For this review, take the finished solid that the model builds, in its own axes (mm). A direction names the side the tool comes from. Coordinates: 2 decimals unless noted, no trailing zeros. Write each loop counter-clockwise with the first axis right and the second up, starting at its lowest first coordinate (ties: lowest second). Pieces come first, ordered by that corner, then holes.
Autodesk Inventor part; units mm, degrees
ref_plane "YZ Plane" through (0, 0, 0) normal (1, 0, 0) x (0, 1, 0)
ref_plane "XZ Plane" through (0, 0, 0) normal (0, 1, 0) x (-1, 0, 0)
ref_plane "XY Plane" through (0, 0, 0) normal (0, 0, 1) x (1, 0, 0)
sketch "Szkic1" plane through (0, 0, 0) normal (0, 1, 0) x (-1, 0, 0)
  circle A0 centre (0, 0) radius 19.62 construction
  line L0 (0, 0) -> (-19.62, 0) construction
  circle A1 centre (0, 0) radius 22.5 construction
  circle A2 centre (-19.3219, 3.407) radius 1.75
  circle A3 centre (-19.3219, -3.407) radius 1.75
  circle A4 centre (6.7104, 18.4368) radius 1.75
  circle A5 centre (12.6115, 15.0298) radius 1.75
  circle A6 centre (12.6115, -15.0298) radius 1.75
  circle A7 centre (6.7104, -18.4368) radius 1.75
  circle A8 centre (0, 0) radius 35
  circle A9 centre (-19.3219, 3.407) radius 3.25
  circle A10 centre (-19.3219, -3.407) radius 3.25
  circle A11 centre (6.7104, -18.4368) radius 3.25
  circle A12 centre (12.6115, -15.0298) radius 3.25
  circle A13 centre (12.6115, 15.0298) radius 3.25
  circle A14 centre (6.7104, 18.4368) radius 3.25
  line L1 (14.2365, 17.8444) -> (8.3354, 21.2514)
  line L2 (10.9865, 12.2152) -> (5.0854, 15.6222)
  line L3 (-16.0719, 3.407) -> (-16.0719, -3.407)
  line L4 (14.2365, -17.8444) -> (8.3354, -21.2514)
  line L5 (10.9865, -12.2152) -> (5.0854, -15.6222)
  line L6 (-22.5719, -3.407) -> (-22.5719, 3.407)
  line L7 (-40, 35) -> (40, 35)
  line L8 (40, 35) -> (40, -35)
  line L9 (40, -35) -> (-40, -35)
  line L10 (-40, -35) -> (-40, 35)
  line L11 (-40, 35) -> (40, -35) construction
  line L12 (40, 35) -> (-40, -35) construction
  line L13 (0, -35) -> (0, 35)
  line L14 (40, 0) -> (-40, 0)
  line L15 (56, 0) -> (-56, 0)
  point P0 (0, -35)
  point P1 (0, 35)
  point P2 (35, 0)
  point P3 (-35, 0)
  dimension "d0" = 39.24
  dimension "d1" = 3.5
  dimension "d2" = 20
  dimension "d5" = 360
  dimension "d7" = 45
  dimension "d8" = 70
  dimension "d12" = 6.5
  dimension "d15" = 360
  dimension "d27" = 80
  dimension "d28" = 70
revolve "Obrót2" add sketch "Szkic1" angle 180 about axis through (-10, 0, 0) along (-1, 0, 0) picked at (16.0586, 3.9431) contours A2 | A4 | A5 | L14 L13 A8 | A8 L7 L8 L14 | L13 L14 L3 A9 L6 A8 | A8 L14 L10 L7 | L14 L6 A9 L3 | A9 | A13 | A13 L2 A14 L1 | A14
extrude "Wyciągnięcie proste1" cut sketch "Szkic1" along normal through all contours A2 | A3 | A4 | A5 | A6 | A7 | L14 L6 A9 L3 | L3 A10 L6 L14 | A9 | A10 | A11 | A11 L5 A12 L4 | A12 | A13 | A13 L2 A14 L1 | A14
extrude "Wyciągnięcie proste2" add sketch "Szkic1" along normal blind 17.85 contours L14 L6 A9 L3 | L3 A10 L6 L14 | A9 | A10 | A11 | A11 L5 A12 L4 | A12 | A13 | A13 L2 A14 L1 | A14
extrude "Wyciągnięcie proste3" cut sketch "Szkic1" along normal blind 7.85 contours A2 | A3 | A4 | A5 | A6 | A7 | L14 L13 A8 | L14 L8 L9 A8 | A8 L7 L8 L14 | A8 L13 L14 | L13 L14 L3 A9 L6 A8 | A8 L14 L10 L7 | L9 L10 L14 A8 | A8 L14 L6 A10 L3 L13 | L14 L6 A9 L3 | L3 A10 L6 L14 | A9 | A10 | A11 | A11 L5 A12 L4 | A12 | A13 | A13 L2 A14 L1 | A14
fillet "Zaokrąglenie1" radius 2 2 edges at (-40, 35, 0) (40, 35, 0)
properties part number "semicylinder_1"
Q1. Clearance check with flat-ended pins moving along their axes: pin 1 Ø3 at (x, z) = (-11, -14.5) entering from +Y; pin 2 Ø3 at (x, z) = (-26.5, 14.5) entering from +Y; pin 3 Ø4 at (x, z) = (19.5, 21) entering from +Y; pin 4 Ø2 at (x, z) = (19.32, -3.41) entering from -Y. State where each tip first meets the part, or that it passes through.
Ans:
pin 1: stops at y = 17.85
pin 2: stops at y = 32.5
pin 3: stops at y = 29.39
pin 4: passes through
Q2. For probe 1 along X at (y, z) = (10.5, 3.5); probe 2 along Z at (x, y) = (-14, 14.75); probe 3 along X at (y, z) = (26, -1), list the stretches that pass through material, from the lowest coordinate up.
Ans:
probe 1: x = -40 to 17.57, 21.07 to 40
probe 2: z = -31.74 to -16.09, -13.96 to 13.96, 16.09 to 31.74
probe 3: x = -40 to 16.07, 22.57 to 40
Q3. Add section B-B (y = 14). Give the number of separate pieces and of enclosed holes in the cut face, then the cut area to 3 significant figures.
Ans:
separate pieces: 1
enclosed holes: 6
area: 5,070 mm2
Q4. Add section A-A (x = 19). State the section outline as (y, z) points.
Ans:
outline: (7.85, -34.11) arc R35 ccw to (34.36, -6.64) - (17.85, -6.64) - (17.85, -5.13) - (7.85, -5.13) - close; (7.85, -1.69) - (17.85, -1.69) - (17.85, 1.69) - (7.85, 1.69) - close; (7.85, 5.13) - (17.85, 5.13) - (17.85, 6.64) - (34.36, 6.64) arc R35 ccw to (7.85, 34.11) - close
Q5. Tool access review of faces 1 (the flat face through (19, 17.85, 0)), 2 (the flat face through (1, 7.85, 0)): name each direction out of +Z, -Z, +X, -X, +Y, -Y from which nothing blocks a thin tool from reaching the whole face with its end or side.
Ans:
face 1: +Y
face 2: +Z, -Z, +X, -X, -Y
Q6. Draft analysis for pull direction X (two halves, no side actions). For faces 3 (the flat face through (-40, 18, 0)), 4 (the flat face through (-11.327, 23.894, 19.524)), 5 (the flat face through (40, 18, 0)), state which applies: +X half, -X half, draft (parallel to the pull), parting line (faces both ways), or undercut.
Ans:
face 3: -X half
face 4: undercut
face 5: +X half
Q7. Add section C-C (x = 10.5). State the section outline as (y, z) points, then the cut area to 3 significant figures.
Ans:
outline: (7.85, -34.11) arc R35 ccw to (7.85, 34.11) - close
area: 1,380 mm2
